from build123d import *

# Parameters (mm, degrees)
F0_W     = 18.75
F0_H     = 12.65
F0_W_2   = 16.75
F0_H_2   = 10.65
F1_DEPTH = 3
F2_W     = 20.8
F2_H     = 16.3
F2_W_2   = 18.75
F2_H_2   = 12.65
F2_W_3   = 16.75
F2_H_3   = 10.65
F3_DEPTH = 9
F4_SIZE  = 1
F5_SIZE  = 0.5


with BuildPart() as f1:
    # F0 (on Front) → F1 (new body)
    with BuildSketch(Plane.XZ):
        with Locations((-53.0061718459, 27.9083168134)):
            Rectangle(F0_W, F0_H)
        with Locations((-53.0061718459, 27.9083168134)):
            Rectangle(F0_W_2, F0_H_2, mode=Mode.SUBTRACT)
    extrude(amount=F1_DEPTH)

    # F2 (on face) → F3 (join)
    with BuildSketch(Plane.XZ.offset(3)):
        with Locations((-53.0061718459, 27.9083168134)):
            Rectangle(F2_W, F2_H)
        with Locations((-53.0061718459, 27.9083168134)):
            Rectangle(F2_W_2, F2_H_2, mode=Mode.SUBTRACT)
        with Locations((-53.0061718459, 27.9083168134)):
            Rectangle(F2_W_2, F2_H_2)
        with Locations((-53.0061718459, 27.9083168134)):
            Rectangle(F2_W_3, F2_H_3, mode=Mode.SUBTRACT)
    extrude(amount=F3_DEPTH)

    # F4
    f4_edges = [f1.edges().sort_by_distance(p)[0] for p in [
        (-53.006172, -12, 33.233317),
        (-44.631172, -12, 27.908317),
        (-53.006172, -12, 22.583317),
        (-61.381172, -12, 27.908317),
    ]]
    chamfer(f4_edges, length=F4_SIZE)

    # F5
    f5_edges = [f1.edges().sort_by_distance(p)[0] for p in [
        (-53.006172, 0, 34.233317),
        (-62.381172, 0, 27.908317),
        (-53.006172, 0, 21.583317),
        (-43.631172, 0, 27.908317),
        (-53.006172, -12, 36.058317),
        (-63.406172, -12, 27.908317),
        (-53.006172, -12, 19.758317),
        (-42.606172, -12, 27.908317),
    ]]
    chamfer(f5_edges, length=F5_SIZE)


solid = f1.part
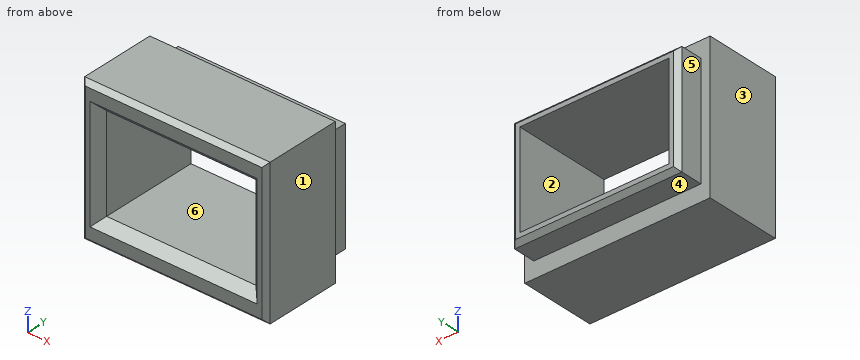
Read the model definition and answer for the solid it produces. Units are mm, in the model's axes. Face numbers are marked on the shaded views. A direction names the side the tool comes from. Coordinates: 2 decimals unless noted, no trailing zeros. Loops run counter-clockwise (first coordinate to the right, second up) from the corner with the lowest first, then second, coordinate; pieces in that order, holes last.
Q1. Each of these flat-tipped pins is pushed along its axis until it touches: pin 1 Ø1.2 at (x, y) = (-53.5, -1) entering from +Z; pin 2 Ø1.2 at (x, y) = (-57, -2) entering from -Z. Where does it stop, or does it pass through?
Q2. Consider probe 1 along X at (y, z) = (-6.25, 32.5); probe 2 along Z at (x, y) = (-46.5, -9.75); probe 3 along X at (y, z) = (-1, 29.75). Determine where each line is inside the solid, lowest interval first.
Q3. Which of the six approach directions +Z, -Z, +X, -X, +Y, -Y give full straight-line access (tool end or side, diameter ignored) to the marked faces 4, 5 and 6?
Q4. The part is cut by section C-C on y = -2.75. Write down the section's boundary in (x, z), and give its area (3 significant figures).
Q5. The part is cut by section D-D on z = 34.5. Write down the section's boundary in (x, y), and give its area (3 significant figures).
Q6. The mould has two halves that part along X. Classify the marked faces 1, 2 and 3: +X half, -X half, draft (parallel to the pull), parting line (faces both ways), or undercut.
Q7. The part is cut by section B-B on z = 30.5. Write down the section's boundary in (x, y), and give its area (4 significant figures).
Q8. The part is cut by section A-A on x = -52. Write down the section's boundary in (y, z), and give its area (4 significant figures).
Results below:
1. pin 1: stops at z = 34.23
1. pin 2: stops at z = 21.58
2. probe 1: x = -63.41 to -61.38, -44.63 to -42.61
2. probe 2: z = 19.76 to 22.58, 33.23 to 36.06
2. probe 3: x = -62.38 to -61.38, -44.63 to -43.63
3. face 4: -Z, +X, -X, +Y
3. face 5: +Z, -Z, -X, +Y
3. face 6: +Y, -Y
4. outline: (-62.38, 21.58) - (-43.63, 21.58) - (-43.63, 34.23) - (-62.38, 34.23) - close; hole (-61.38, 22.58) - (-44.63, 22.58) - (-44.63, 33.23) - (-61.38, 33.23) - close
4. area: 58.8 mm2
5. outline: (-63.41, -11.5) - (-62.91, -12) - (-43.11, -12) - (-42.61, -11.5) - (-42.61, -3) - (-63.41, -3) - close
5. area: 187 mm2
6. face 1: +X half
6. face 2: undercut
6. face 3: -X half
7. outline: (-63.41, -11.5) - (-62.91, -12) - (-62.38, -12) - (-61.38, -11) - (-61.38, 0) - (-61.88, 0) - (-62.38, -0.5) - (-62.38, -3) - (-63.41, -3) - close; (-44.63, -11) - (-43.63, -12) - (-43.11, -12) - (-42.61, -11.5) - (-42.61, -3) - (-43.63, -3) - (-43.63, -0.5) - (-44.13, 0) - (-44.63, 0) - close
7. area: 40.95 mm2
8. outline: (-12, 20.26) - (-11.5, 19.76) - (-3, 19.76) - (-3, 21.58) - (-0.5, 21.58) - (0, 22.08) - (0, 22.58) - (-11, 22.58) - (-12, 21.58) - close; (-12, 34.23) - (-11, 33.23) - (0, 33.23) - (0, 33.73) - (-0.5, 34.23) - (-3, 34.23) - (-3, 36.06) - (-11.5, 36.06) - (-12, 35.56) - close
8. area: 55.35 mm2
